```python
from build123d import *

# Parameters (mm, degrees)
BOSS_EXTRUDE1_DEPTH = 13.5
SKETCH2_R           = 2.5
BOSS_EXTRUDE2_DEPTH = 2.5


with BuildPart() as part:
    # Sketch1 → Boss-Extrude1 (new body)
    with BuildSketch(Plane(origin=(0, 0, 0), x_dir=(1, 0, 0), z_dir=(0, 1, 0))):
        Polygon((30.066607979, 23.493934911), (30.066607979, 4.493934911), (38.066607979, 4.493934911), (38.066607979, 23.493934911), (41.066607979, 23.493934911), (41.066607979, 29.493934911), (53.066607979, 29.493934911), (53.066607979, 37.993934911), (55.066607979, 37.993934911), (55.066607979, 42.993934911), (53.066607979, 42.993934911), (53.066607979, 45.993934911), (48.566607979, 45.993934911), (48.566607979, 54.593934911), (43.066607979, 54.593934911), (25.066607979, 54.593934911), (19.566607979, 54.593934911), (19.566607979, 45.993934911), (15.066607979, 45.993934911), (15.066607979, 42.993934911), (13.066607979, 42.993934911), (13.066607979, 37.993934911), (15.066607979, 37.993934911), (15.066607979, 29.493934911), (27.066607979, 29.493934911), (27.066607979, 23.493934911), align=None)
    extrude(amount=BOSS_EXTRUDE1_DEPTH)

    # Sketch2 → Boss-Extrude2 (add)
    with BuildSketch(Plane.XZ):
        with Locations((34.066607979, -32.993934911)):
            Circle(SKETCH2_R)
    extrude(amount=BOSS_EXTRUDE2_DEPTH)


solid = part.part
```
Geometry check sheet. Reference: the model listing, model coordinates, mm. A direction names the side the tool comes from. Give positions to 0.01 mm unless a question says otherwise; leave off trailing zeros. Order: outer loops, then holes, each group sorted by start corner. A loop starts at its lowest first (then second) coordinate and runs counter-clockwise, first axis right, second up. Notation, with made-up numbers: (79, 15) - (99, 15) arc R14 ccw to (99, 32) - close; hole circle Ø8 at (0, -24.75). An arc over 180 degrees is marked (long way). Answer in a Markdown table with one row per item. Add a question column.
Q1. Cross-section at A-A, the plane y = 4.75. Enter the section's corners in (x, z), then the cut area to 3 significant figures.
Q2. Material ranges on probe 1 along Y at (x, z) = (31, -12); probe 2 along X at (y, z) = (10.25, -8.5); probe 3 along X at (y, z) = (-0.5, -33), recorded low to high. Write a range as from..to.
Q3. Cross-section at D-D, the plane z = -20.5. Enter the section's corners in (x, y).
Q4. Cross-section at C-C, the plane z = -51. Enter the section's corners in (x, y).
Q5. Cross-section at B-B, the plane x = 34. Enter the section's corners in (y, z), then the cut area to 3 significant figures.
Q6. Gauge pin test, flat ends, axial feed: pin 1 (1 mm diameter, centred on x = 14.5, y = 9, fed in from -Z); pin 2 (1.5 mm diameter, centred on y = 4, z = -44, fed in from +X); pin 3 (8 mm diameter, centred on x = 38.5, z = -11, fed in from -Y); pin 4 (3.5 mm diameter, centred on y = 8, z = -44.5, fed in from -X). Record the tip position at first contact, or that the pin passes through.
Q7. Tool access check on faces 1 (the flat face through (41.067, 7, -26)), 2 (the flat face through (19.567, 7, -50)), 3 (the flat face through (51, 7, -45.994)), 4 (the flat face through (27.067, 7, -27)). Record the directions out of +Z, -Z, +X, -X, +Y, -Y that give a thin tool (end or side, any length) a straight path to the whole face; none if there is none.
Check values:
| question | item | result |
|---|---|---|
| 1 | outline | (13.07, -42.99) - (15.07, -42.99) - (15.07, -45.99) - (19.57, -45.99) - (19.57, -54.59) - (48.57, -54.59) - (48.57, -45.99) - (53.07, -45.99) - (53.07, -42.99) - (55.07, -42.99) - (55.07, -37.99) - (53.07, -37.99) - (53.07, -29.49) - (41.07, -29.49) - (41.07, -23.49) - (38.07, -23.49) - (38.07, -4.49) - (30.07, -4.49) - (30.07, -23.49) - (27.07, -23.49) - (27.07, -29.49) - (15.07, -29.49) - (15.07, -37.99) - (13.07, -37.99) - close |
| 1 | area | 1,130 mm^2 |
| 2 | probe 1 | y = 0..13.5 |
| 2 | probe 2 | x = 30.07..38.07 |
| 2 | probe 3 | x = 31.57..36.57 |
| 3 | outline | (30.07, 0) - (38.07, 0) - (38.07, 13.5) - (30.07, 13.5) - close |
| 4 | outline | (19.57, 0) - (48.57, 0) - (48.57, 13.5) - (19.57, 13.5) - close |
| 5 | outline | (-2.5, -35.49) - (0, -35.49) - (0, -54.59) - (13.5, -54.59) - (13.5, -4.49) - (0, -4.49) - (0, -30.49) - (-2.5, -30.49) - close |
| 5 | area | 689 mm^2 |
| 6 | pin 1 | stops at z = -42.99 |
| 6 | pin 2 | stops at x = 53.07 |
| 6 | pin 3 | stops at y = 0 |
| 6 | pin 4 | stops at x = 13.07 |
| 7 | face 1 | +Z, +X, +Y, -Y |
| 7 | face 2 | -Z, -X, +Y, -Y |
| 7 | face 3 | -Z, +X, +Y, -Y |
| 7 | face 4 | +Z, -X, +Y, -Y |
